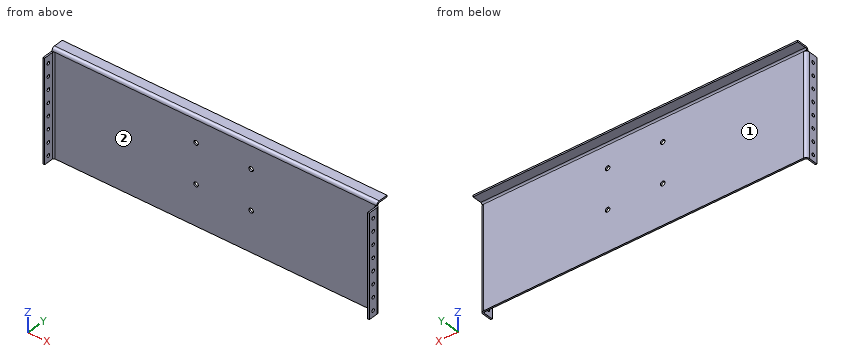
```python
from build123d import *

# Parameters (mm, degrees)
SKETCH1_W                    = 489.688000048
SKETCH1_H                    = 177.8
BASE_FLANGE1_DEPTH           = 2.3622
EDGE_FLANGE1_STRIP_W         = 14.1688
EDGE_FLANGE1_STRIP_H         = 2.3622
EDGE_FLANGE1_STRIP_CUT_DEPTH = 489.688000048
EDGE_FLANGE1_DEPTH           = 489.688000048
EDGE_FLANGE2_STRIP_W         = 14.1688
EDGE_FLANGE2_STRIP_H         = 2.3622
EDGE_FLANGE2_STRIP_CUT_DEPTH = 173.0778
EDGE_FLANGE2_DEPTH           = 173.0778
EDGE_FLANGE3_STRIP_W         = 14.1688
EDGE_FLANGE3_STRIP_H         = 2.3622
EDGE_FLANGE3_STRIP_CUT_DEPTH = 173.0778
EDGE_FLANGE3_DEPTH           = 173.0778
SKETCH15_R                   = 3.4
CUT_EXTRUDE1_DEPTH           = 6.35
SKETCH33_W                   = 534.836919658
SKETCH33_H                   = 38.1
CUT_EXTRUDE5_DEPTH           = 264.395174273
SKETCH37_R                   = 2.413
CUT_EXTRUDE8_DEPTH           = 501.379367947


# Sheet-metal steps are written as plain solids
with BuildPart() as part:
    # Sketch1 → Base-Flange1 (new body)
    with BuildSketch(Plane(origin=(0, 0, 0), x_dir=(1, 0, 0), z_dir=(0, 1, 0))):
        Rectangle(SKETCH1_W, SKETCH1_H)
    extrude(amount=-BASE_FLANGE1_DEPTH)

    # Edge-Flange1 strip (across the edge) → Edge-Flange1 strip cut (cut)
    with BuildSketch(Plane(origin=(-244.844000024, 0, 88.9), x_dir=(0, 0, -1), z_dir=(1, 0, 0))):
        with Locations((-2.3622, -1.1811)):
            Rectangle(EDGE_FLANGE1_STRIP_W, EDGE_FLANGE1_STRIP_H)
    extrude(amount=EDGE_FLANGE1_STRIP_CUT_DEPTH, mode=Mode.SUBTRACT)

    # Edge-Flange1 section (across the edge) → Edge-Flange1 (add)
    with BuildSketch(Plane(origin=(-244.844000024, 0, 88.9), x_dir=(0, 0, -1), z_dir=(1, 0, 0))):
        with BuildLine():
            Line((0, 2.36), (0, 16.6878))
            Line((0, 16.6878), (2.3622, 16.6878))
            Line((2.3622, 16.6878), (2.3622, 2.36))
            ThreePointArc((2.3622, 2.36), (3.053427996, 0.691227996), (4.7222, 0))
            Line((4.7222, 0), (4.7222, -2.3622))
            ThreePointArc((4.7222, -2.3622), (1.383100358, -0.979099642), (0, 2.36))
        make_face()
    extrude(amount=EDGE_FLANGE1_DEPTH)

    # Edge-Flange2 strip (across the edge) → Edge-Flange2 strip cut (cut)
    with BuildSketch(Plane(origin=(-244.844000024, -2.3622, 84.1778), x_dir=(1, 0, 0), z_dir=(0, 0, -1))):
        with Locations((-2.3622, -1.1811)):
            Rectangle(EDGE_FLANGE2_STRIP_W, EDGE_FLANGE2_STRIP_H)
    extrude(amount=EDGE_FLANGE2_STRIP_CUT_DEPTH, mode=Mode.SUBTRACT)

    # Edge-Flange2 section (across the edge) → Edge-Flange2 (add)
    with BuildSketch(Plane(origin=(-244.844000024, -2.3622, 84.1778), x_dir=(1, 0, 0), z_dir=(0, 0, -1))):
        with BuildLine():
            Line((0, 2.36), (0, 16.6878))
            Line((0, 16.6878), (2.3622, 16.6878))
            Line((2.3622, 16.6878), (2.3622, 2.36))
            ThreePointArc((2.3622, 2.36), (3.053427996, 0.691227996), (4.7222, 0))
            Line((4.7222, 0), (4.7222, -2.3622))
            ThreePointArc((4.7222, -2.3622), (1.383100358, -0.979099642), (0, 2.36))
        make_face()
    extrude(amount=EDGE_FLANGE2_DEPTH)

    # Edge-Flange3 strip (across the edge) → Edge-Flange3 strip cut (cut)
    with BuildSketch(Plane(origin=(244.844000024, -2.3622, -88.9), x_dir=(-1, 0, 0), z_dir=(0, 0, 1))):
        with Locations((-4.7244, -1.1811)):
            Rectangle(EDGE_FLANGE3_STRIP_W, EDGE_FLANGE3_STRIP_H)
    extrude(amount=EDGE_FLANGE3_STRIP_CUT_DEPTH, mode=Mode.SUBTRACT)

    # Edge-Flange3 section (across the edge) → Edge-Flange3 (add)
    with BuildSketch(Plane(origin=(244.844000024, -2.3622, -88.9), x_dir=(-1, 0, 0), z_dir=(0, 0, 1))):
        with BuildLine():
            Line((-2.3622, 2.36), (-2.3622, 16.6878))
            Line((-2.3622, 16.6878), (0, 16.6878))
            Line((0, 16.6878), (0, 2.36))
            ThreePointArc((0, 2.36), (0.691227996, 0.691227996), (2.36, 0))
            Line((2.36, 0), (2.36, -2.3622))
            ThreePointArc((2.36, -2.3622), (-0.979099642, -0.979099642), (-2.3622, 2.36))
        make_face()
    extrude(amount=EDGE_FLANGE3_DEPTH)

    # Sketch15 → Cut-Extrude1 (cut)
    with BuildSketch(Plane(origin=(0, 0, 0), x_dir=(1, 0, 0), z_dir=(0, 1, 0))):
        with Locations(Location((-27.621800024, 9.3222, 0), (0, 0, 270))):
            Circle(SKETCH15_R)
        with Locations(Location((-27.621800024, -50.6778, 0), (0, 0, 270))):
            Circle(SKETCH15_R)
        with Locations(Location((55.378199976, 9.3222, 0), (0, 0, 270))):
            Circle(SKETCH15_R)
        with Locations(Location((55.378199976, -50.6778, 0), (0, 0, 270))):
            Circle(SKETCH15_R)
    extrude(amount=-CUT_EXTRUDE1_DEPTH, mode=Mode.SUBTRACT)

    # Sketch33 → Cut-Extrude5 (cut, through all)
    with BuildSketch(Plane(origin=(0, 0, 0), x_dir=(1, 0, 0), z_dir=(0, 1, 0))):
        with Locations((1.1811, 88.9)):
            Rectangle(SKETCH33_W, SKETCH33_H)
    extrude(amount=-CUT_EXTRUDE5_DEPTH, mode=Mode.SUBTRACT)

    # Sketch37 → Cut-Extrude8 (cut, through all)
    with BuildSketch(Plane.ZY.offset(244.844000024)):
        with Locations(Location((72.824, -11.8861, 0), (0, 0, 270))):
            Circle(SKETCH37_R)
        with Locations(Location((53.774, -11.8861, 0), (0, 0, 270))):
            Circle(SKETCH37_R)
        with Locations(Location((34.724, -11.8861, 0), (0, 0, 270))):
            Circle(SKETCH37_R)
        with Locations(Location((15.674, -11.8861, 0), (0, 0, 270))):
            Circle(SKETCH37_R)
        with Locations(Location((-3.376, -11.8861, 0), (0, 0, 270))):
            Circle(SKETCH37_R)
        with Locations(Location((-22.426, -11.8861, 0), (0, 0, 270))):
            Circle(SKETCH37_R)
        with Locations(Location((-41.476, -11.8861, 0), (0, 0, 270))):
            Circle(SKETCH37_R)
        with Locations(Location((-60.526, -11.8861, 0), (0, 0, 270))):
            Circle(SKETCH37_R)
    extrude(amount=-CUT_EXTRUDE8_DEPTH, mode=Mode.SUBTRACT)


solid = part.part
```
Geometry check sheet. Reference: the model listing, model coordinates, mm. Face numbers are marked on the shaded views. Coordinates: 2 decimals unless noted, no trailing zeros. Write each loop counter-clockwise with the first axis right and the second up, starting at its lowest first coordinate (ties: lowest second). Pieces come first, ordered by that corner, then holes. Notation, with made-up numbers: M 61.25,8.25 L 119.25,8.25 A9 cw 119.25,23.25 Z; hole C -12,19.25 d1. An arc over 180 degrees is marked long. Answer as a JSON object with one key per item and string values.
1. Draft check along X on the marked faces 1 and 2. Enter one of: released by +X, released by -X, zero draft, split by the parting line, or undercut.
Answers below:
{"face 1": "zero draft", "face 2": "undercut"}
2. Go/stop test with flat-tipped pins: pin 1 Ø11 at (x, z) = (-27.62, -9.32) entering from -Y; pin 2 Ø7.5 at (y, z) = (-11.89, -3.38) entering from -X; pin 3 Ø3 at (x, z) = (-36, 37.5) entering from +Y; pin 4 Ø12 at (y, z) = (5, 43) entering from -X. Record where each tip stops, or that it passes through.
Answers below:
{"pin 1": "stops at y = -2.36", "pin 2": "stops at x = -244.84", "pin 3": "stops at y = 0", "pin 4": "stops at x = -243.03"}
3. Section check A-A, the plane z = 3.5. Enter the section's corners in (x, y), plus the area to 3 significant figures.
Answers below:
{"outline": "M -244.84,-19.05 L -242.48,-19.05 L -242.48,-4.72 A2.36 cw -240.12,-2.36 L 242.48,-2.36 A2.36 cw 244.84,-4.72 L 244.84,-19.05 L 247.21,-19.05 L 247.21,-4.72 A4.72 ccw 242.48,0 L -240.12,0 A4.72 ccw -244.84,-4.72 Z", "area": "1,230 mm²"}
4. Section check C-C, the plane y = 11.5. Enter the section's corners in (x, z), plus the area to 3 significant figures.
Answers below:
{"outline": "M -244.84,86.54 L 244.84,86.54 L 244.84,88.9 L -244.84,88.9 Z", "area": "1,160 mm²"}
5. Scan lines: L1, parallel to X at y = -5, z = -27.5; L2, parallel to Y at x = 142.5, z = -25.5; L3, parallel to Z at x = 18, y = 7. Record each from-to range of solid material in increasing order.
Answers below:
{"L1": "x = -244.84 to -242.48, 244.84 to 247.21", "L2": "y = -2.36 to 0", "L3": "z = 86.54 to 88.9"}
6. Section check B-B, the plane x = -177. Enter the section's corners in (y, z).
Answers below:
{"outline": "M -2.36,-69.85 L 0,-69.85 L 0,84.18 A2.36 cw 2.36,86.54 L 16.69,86.54 L 16.69,88.9 L 2.36,88.9 A4.72 ccw -2.36,84.18 Z"}
